Input: dimensioned drawing with shaded views. Units: mm. Origin: part minimum x, y, z. Coordinates: 2 decimals unless noted, no trailing zeros. One line per question, with ' | ' between items. Start each with the question number.
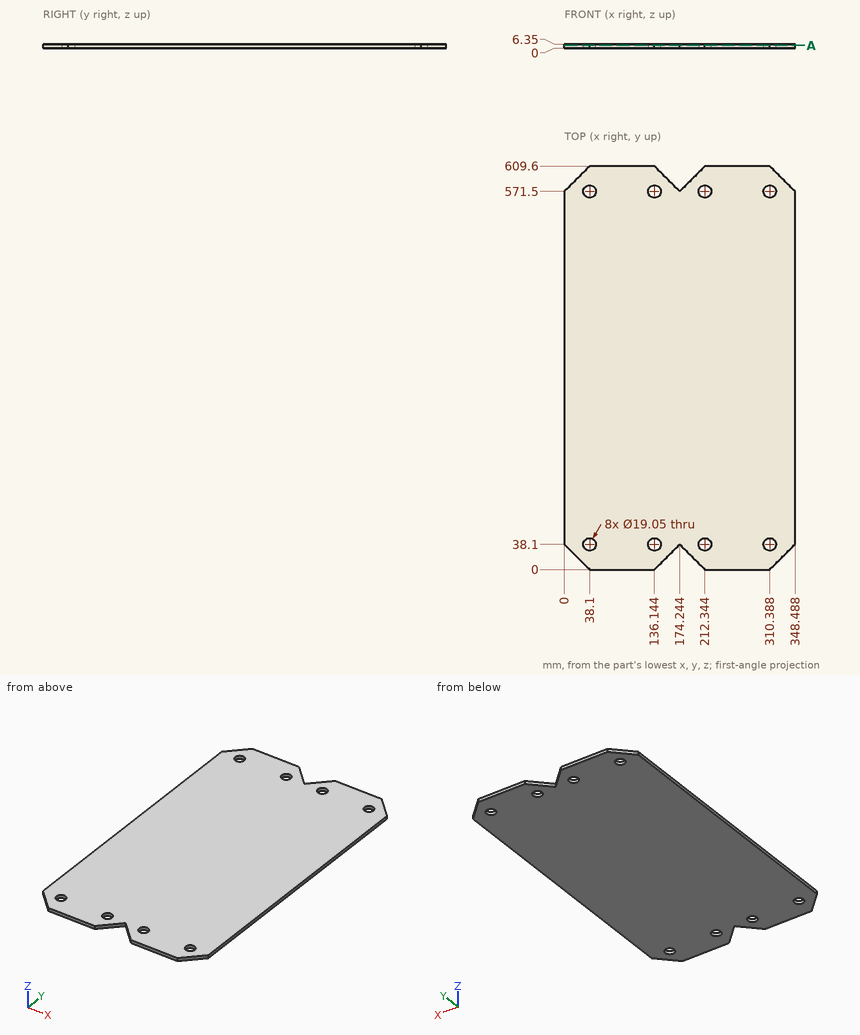
(1) Material intervals for line 1 along Y through (x, z) = (41, 4.5); line 2 along Y through (x, z) = (319, 3.5); line 3 along Y through (x, z) = (167.5, 0.5), sorted ascending. Write a range as from..to.
(2) Section A-A (z = 4.25). State how many separate pieces and enclosed holes the cut face has, then the cut area to 3 significant figures.
(3) Pin query (flat end, axial travel): pin 1 (22 mm diameter, centred on x = 212.344, y = 38.1, fed in from -Z); pin 2 (11.5 mm diameter, centred on x = 38.1, y = 571.5, fed in from -Z). Return the tip coordinate at first contact, or that it passes through.
Worked answers:
1) line 1: y = 0..29.03, 47.17..562.43, 580.57..609.6 | line 2: y = 8.61..34.03, 42.17..567.43, 575.57..600.99 | line 3: y = 31.36..578.24
2) separate pieces: 1 | enclosed holes: 8 | area: 204,000 mm²
3) pin 1: stops at z = 0 | pin 2: passes through
